Geometry check sheet. Reference: the model listing, model coordinates, mm. A direction names the side the tool comes from. Give positions to 0.01 mm unless a question says otherwise; leave off trailing zeros. Loops run counter-clockwise (first coordinate to the right, second up) from the corner with the lowest first, then second, coordinate; pieces in that order, holes last. Notation, with made-up numbers: (-38, 51) -> (-24, 51) arc R19 ccw to (-24, 65) -> close; hole circle Ø10 at (80.25, -15). An arc over 180 degrees is marked (long way). Write item = value, one per line. Start each with the question number.
```python
from build123d import *

# Parameters (mm, degrees)
SKETCH1_W                = 86
SKETCH1_H                = 60
BOSS_EXTRUDE1_DEPTH      = 6
M5_CLEARANCE_HOLE1_D     = 5.3
FILLET1_R                = 10
M5_CLEARANCE_HOLE2_D     = 5.3
F_8_0_8_DIAMETER_HOLE1_D = 8
M3_CLEARANCE_HOLE1_D     = 3.2
SKETCH6_R                = 11
CUT_EXTRUDE3_DEPTH       = 7
FILLET1343_R             = 1
SKETCH73_W               = 6.1
SKETCH73_H               = 10.1
CUT_EXTRUDE24_DEPTH      = 4
CUT_EXTRUDE24_DEPTH_BACK = 4
SKETCH74_W               = 6.1
SKETCH74_H               = 10.1
CUT_EXTRUDE25_DEPTH      = 4
CUT_EXTRUDE25_DEPTH_BACK = 4
SKETCH2349_W             = 10
SKETCH2349_H             = 6
BOSS_EXTRUDE2347_DEPTH   = 6
FILLET1346_R             = 1


with BuildPart() as part:
    # Sketch1 → Boss-Extrude1 (new body)
    with BuildSketch(Plane(origin=(0, 0, 0), x_dir=(1, 0, 0), z_dir=(0, 1, 0))):
        Rectangle(SKETCH1_W, SKETCH1_H)
    extrude(amount=BOSS_EXTRUDE1_DEPTH)

    # M5 Clearance Hole1 (through all)
    with Locations(Plane(origin=(0, 6, 0), x_dir=(1, 0, 0), z_dir=(0, 1, 0))):
        with Locations((-35.6, 0)):
            Hole(M5_CLEARANCE_HOLE1_D / 2)

    # Fillet1
    fillet1_edges = [part.edges().sort_by_distance(p)[0] for p in [
        (43, 3, -30),
    ]]
    fillet(fillet1_edges, radius=FILLET1_R)

    # M5 Clearance Hole2 (through all)
    with Locations(Plane(origin=(0, 6, 0), x_dir=(1, 0, 0), z_dir=(0, 1, 0))):
        with Locations((37, 0)):
            Hole(M5_CLEARANCE_HOLE2_D / 2)

    # 8.0 _8_ Diameter Hole1 (through all)
    with Locations(Plane(origin=(0, 6, 0), x_dir=(1, 0, 0), z_dir=(0, 1, 0))):
        with Locations((23.4, 5)):
            Hole(F_8_0_8_DIAMETER_HOLE1_D / 2)

    # M3 Clearance Hole1 (through all)
    with Locations(Plane(origin=(-7.6, 0, -5), x_dir=(1, 0, 0), z_dir=(0, -1, 0))):
        with Locations((15.5, -15.5), (-15.5, -15.5), (-15.5, 15.5), (15.5, 15.5)):
            Hole(M3_CLEARANCE_HOLE1_D / 2)

    # Sketch6 → Cut-Extrude3 (cut, through all)
    with BuildSketch(Plane(origin=(-7.6, 0, -5), x_dir=(-1, 0, 0), z_dir=(0, -1, 0))):
        Circle(SKETCH6_R)
    extrude(amount=-CUT_EXTRUDE3_DEPTH, mode=Mode.SUBTRACT)

    # Fillet1343
    fillet1343_edges = [part.edges().sort_by_distance(p)[0] for p in [
        (-43, 3, -30),
    ]]
    fillet(fillet1343_edges, radius=FILLET1343_R)

    # Sketch73 → Cut-Extrude24 (cut, two sides)
    with BuildSketch(Plane(origin=(8.4, 3, -20), x_dir=(-1, 0, 0), z_dir=(0, -1, 0))) as cut_extrude24_sk:
        with Locations((44, -32.5)):
            Rectangle(SKETCH73_W, SKETCH73_H)
        with Locations((44, -7.5)):
            Rectangle(SKETCH73_W, SKETCH73_H)
    extrude(amount=CUT_EXTRUDE24_DEPTH, mode=Mode.SUBTRACT)
    extrude(cut_extrude24_sk.sketch, amount=-CUT_EXTRUDE24_DEPTH_BACK, mode=Mode.SUBTRACT)

    # Sketch74 → Cut-Extrude25 (cut, two sides)
    with BuildSketch(Plane(origin=(-7, 3, 20), x_dir=(1, 0, 0), z_dir=(0, -1, 0))) as cut_extrude25_sk:
        with Locations((44, -32.5)):
            Rectangle(SKETCH74_W, SKETCH74_H)
        with Locations((44, -7.5)):
            Rectangle(SKETCH74_W, SKETCH74_H)
    extrude(amount=CUT_EXTRUDE25_DEPTH, mode=Mode.SUBTRACT)
    extrude(cut_extrude25_sk.sketch, amount=-CUT_EXTRUDE25_DEPTH_BACK, mode=Mode.SUBTRACT)

    # Sketch2349 → Boss-Extrude2347 (add)
    with BuildSketch(Plane(origin=(8.767778608, 6, 30), x_dir=(-1, 0, 0), z_dir=(0, 0, 1))):
        with Locations((0.767778608, 3)):
            Rectangle(SKETCH2349_W, SKETCH2349_H)
    extrude(amount=BOSS_EXTRUDE2347_DEPTH)

    # Fillet1346
    fillet1346_edges = [part.edges().sort_by_distance(p)[0] for p in [
        (13, 3, 36),
        (3, 3, 36),
    ]]
    fillet(fillet1346_edges, radius=FILLET1346_R)


solid = part.part
```
1) Section check A-A (z = 14). Enter the section's corners in (x, y).
2) Tool access check on faces 4 (the flat face through (-38.65, 3, 13)), 5 (the flat face through (43, 3, 5)). Record the directions out of +Z, -Z, +X, -X, +Y, -Y that give a thin tool (end or side, any length) a straight path to the whole face; none if there is none.
3) Draft check along X on faces 1 (the cylindrical face through (39.99, 3.04, -27.15)), 2 (the flat face through (-38.65, 3, -12)), 3 (the flat face through (-20, 3, 30)). Enter one of: released by +X, released by -X, zero draft, split by the parting line, or undercut.
4) Thickness scan on line 1 (Z direction, x = 7.9, y = 3.2); line 2 (Z direction, x = -23.1, y = 2.3); line 3 (Z direction, x = -7.6, y = 4.5). Record the ranges inside material, lowest first.
5) Section check B-B (x = -7.6). Enter the section's corners in (y, z), plus the area to 3 significant figures.
6) Section check D-D (x = -35.6). Enter the section's corners in (y, z), plus the area to 3 significant figures.
7) Section check C-C (x = 7.9). Enter the section's corners in (y, z).
8) Depth check by flat-ended pin: pin 1 Ø2 at (x, z) = (-21, 15) entering from -Y; pin 2 Ø3 at (x, y) = (-36.5, 2) entering from +Z. Enter the tip coordinate at first touch or a pass-through.
Check result:
q1.outline = (-43, 0) -> (-38.65, 0) -> (-38.65, 6) -> (-43, 6) -> close; (-32.55, 0) -> (33.95, 0) -> (33.95, 6) -> (-32.55, 6) -> close; (40.05, 0) -> (43, 0) -> (43, 6) -> (40.05, 6) -> close
q2.face_4 = +Y, -Y
q2.face_5 = +Z, -Z, +X, +Y, -Y
q3.face_1 = released by +X
q3.face_2 = undercut
q3.face_3 = zero draft
q4.line_1 = -30 to -22.1, -18.9 to 8.9, 12.1 to 36
q4.line_2 = -30 to -22.1, -18.9 to 8.9, 12.1 to 30
q4.line_3 = -30 to -16, 6 to 30
q5.outline = (0, -30) -> (6, -30) -> (6, -16) -> (0, -16) -> close; (0, 6) -> (6, 6) -> (6, 30) -> (0, 30) -> close
q5.area = 228 mm2
q6.outline = (0, -30) -> (6, -30) -> (6, -17.55) -> (0, -17.55) -> close; (0, -7.45) -> (6, -7.45) -> (6, -2.65) -> (0, -2.65) -> close; (0, 2.65) -> (6, 2.65) -> (6, 7.45) -> (0, 7.45) -> close; (0, 17.55) -> (6, 17.55) -> (6, 30) -> (0, 30) -> close
q6.area = 207 mm2
q7.outline = (0, -30) -> (6, -30) -> (6, -22.1) -> (0, -22.1) -> close; (0, -18.9) -> (6, -18.9) -> (6, 8.9) -> (0, 8.9) -> close; (0, 12.1) -> (6, 12.1) -> (6, 36) -> (0, 36) -> close
q8.pin_1 = 0
q8.pin_2 = 30
